The model under review builds one solid part; all positions refer to its coordinate system, in mm. Face numbers are marked on the shaded views. A direction names the side the tool comes from. Round coordinates to 2 decimals unless told otherwise and drop trailing zeros. Write each loop counter-clockwise with the first axis right and the second up, starting at its lowest first coordinate (ties: lowest second). Pieces come first, ordered by that corner, then holes. Notation, with made-up numbers: (48, -37.5) -> (66, -37.5) arc R7 cw to (66, -28.5) -> close; hole circle Ø5 at (18.5, 47). An arc over 180 degrees is marked (long way). Answer as a JSON object with one key per item and string values. Group by question number.
1) Machinability: for the marked faces 1, 2 and 3, which of the approach directions +Z, -Z, +X, -X, +Y, -Y give a long, thin tool a straight path to every point of the face, cutting with its end or side? Answer none if there is none.
2) Mouldability with a two-part tool opening along X and no side actions: class the marked faces 4, 5 and 6 as pulls with the +X half, pulls with the -X half, needs draft (parallel to the pull), parting line crosses it, or undercut.
3) We need section A-A, the plane x = 0. Write out the cut boundary in (y, z).
4) We need section D-D, the plane z = 7. Write out the cut boundary in (x, y), then the cut area to 3 significant figures.
5) We need section C-C, the plane y = 6.5. Write out the cut boundary in (x, z).
6) To check wall thickness, follow probe 1 along Y at (x, z) = (0, 14); probe 2 along Z at (x, y) = (9.5, -21); probe 3 along Z at (x, y) = (1, 12). State the ranges of each line that lie inside material, in increasing order. Write a range as [from, to].
7) Insertion check: pin 1 Ø12 at (x, z) = (-10, 5) entering from -Y; pin 2 Ø5 at (x, z) = (19.5, 23.5) entering from +Y; pin 3 Ø12 at (y, z) = (-12, -0.5) entering from +X. Each pin has a flat end and moves straight along its axis. Give the tip position at first contact, or say it passes through.
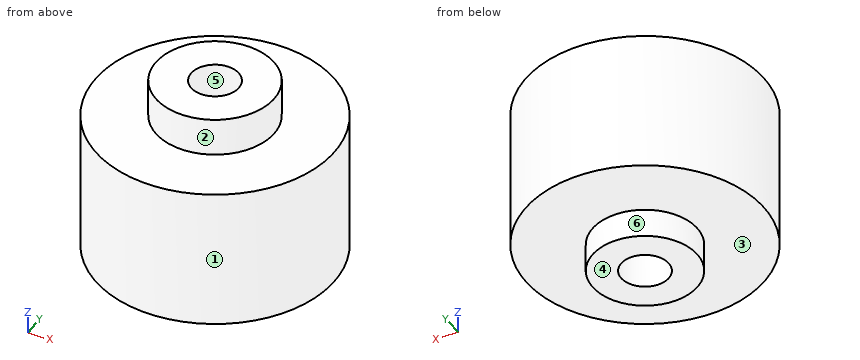
from build123d import *

# Parameters (mm, degrees)
IZIM1_R                     = 25
Y_KSEKLIK_EKSTR_ZYON1_DEPTH = 29.7
IZIM2_R                     = 11
Y_KSEKLIK_EKSTR_ZYON2_DEPTH = 6
IZIM3_R                     = 12.4
Y_KSEKLIK_EKSTR_ZYON3_DEPTH = 8
IZIM4_R                     = 5
KES_EKSTR_ZYON1_DEPTH       = 57.211119896


with BuildPart() as part:
    # Çizim1 → Yükseklik-Ekstrüzyon1 (new body)
    with BuildSketch(Plane.XY):
        Circle(IZIM1_R)
    extrude(amount=Y_KSEKLIK_EKSTR_ZYON1_DEPTH)

    # Çizim2 → Yükseklik-Ekstrüzyon2 (add)
    with BuildSketch(Plane(origin=(0, 0, 0), x_dir=(-1, 0, 0), z_dir=(0, 0, -1))):
        Circle(IZIM2_R)
    extrude(amount=Y_KSEKLIK_EKSTR_ZYON2_DEPTH)

    # Çizim3 → Yükseklik-Ekstrüzyon3 (add)
    with BuildSketch(Plane.XY.offset(29.7)):
        Circle(IZIM3_R)
    extrude(amount=Y_KSEKLIK_EKSTR_ZYON3_DEPTH)

    # Çizim4 → Kes-Ekstrüzyon1 (cut, through all)
    with BuildSketch(Plane.XY.offset(37.7)):
        Circle(IZIM4_R)
    extrude(amount=-KES_EKSTR_ZYON1_DEPTH, mode=Mode.SUBTRACT)


solid = part.part
Here are the results:
{
 "1": {"face 1": "+Z, -Z", "face 2": "+Z", "face 3": "-Z"},
 "2": {"face 4": "needs draft", "face 5": "undercut", "face 6": "parting line crosses it"},
 "3": {"outline": "(-25, 0) -> (-11, 0) -> (-11, -6) -> (-5, -6) -> (-5, 37.7) -> (-12.4, 37.7) -> (-12.4, 29.7) -> (-25, 29.7) -> close; (5, -6) -> (11, -6) -> (11, 0) -> (25, 0) -> (25, 29.7) -> (12.4, 29.7) -> (12.4, 37.7) -> (5, 37.7) -> close"},
 "4": {"outline": "circle Ø50 at (0, 0); hole circle Ø10 at (0, 0)", "area": "1,880 mm^2"},
 "5": {"outline": "(-24.14, 0) -> (-8.87, 0) -> (-8.87, -6) -> (8.87, -6) -> (8.87, 0) -> (24.14, 0) -> (24.14, 29.7) -> (10.56, 29.7) -> (10.56, 37.7) -> (-10.56, 37.7) -> (-10.56, 29.7) -> (-24.14, 29.7) -> close"},
 "6": {"probe 1": "y = [-25, -5], [5, 25]", "probe 2": "z = [0, 29.7]", "probe 3": "z = [0, 37.7]"},
 "7": {"pin 1": "stops at y = -24.68", "pin 2": "stops at y = 18.33", "pin 3": "stops at x = 24.26"}
}
